```python
from build123d import *

# Parameters (mm, degrees)
ESTRUSIONE_ESTRUSIONE1_DEPTH = 2.5
SCHIZZO2_W                   = 10
SCHIZZO2_H                   = 38
ESTRUSIONE_ESTRUSIONE2_DEPTH = 15
SCHIZZO3_W                   = 6
SCHIZZO3_H                   = 33.15
TAGLIO_ESTRUSIONE1_DEPTH     = 20
ESTRUSIONE_SOTTILE1_START    = 19
SCHIZZO5_R                   = 21
SCHIZZO5_R_2                 = 18
ESTRUSIONE_SOTTILE1_DEPTH    = 19
SCHIZZO8_W                   = 38
SCHIZZO8_H                   = 15
TAGLIO_ESTRUSIONE2_DEPTH     = 70.157520353
SCHIZZO10_R                  = 3
ESTRUSIONE_ESTRUSIONE3_DEPTH = 4
FORO_PER_VITE_M1_6_1_D       = 2
FORO_PER_VITE_M1_6_1_DEPTH   = 3
FORO_PER_VITE_M1_6_1_TIP     = 0.600860619
SCHIZZO12_R                  = 1
TAGLIO_ESTRUSIONE3_DEPTH     = 3
FORO_PER_VITE_M3_1_D         = 3.6
FORO_PER_VITE_M3_1_DEPTH     = 4
FORO_PER_VITE_M3_1_TIP       = 1.081549114


with BuildPart() as part:
    # Schizzo1 → Estrusione-Estrusione1 (new, symmetric)
    with BuildSketch(Plane.XY):
        with BuildLine():
            Line((12.36549987, -26.390648792), (47.36549987, -26.390648792))
            Line((47.36549987, -26.390648792), (47.36549987, 11.609351208))
            Line((47.36549987, 11.609351208), (12.36549987, 11.609351208))
            ThreePointArc((12.36549987, 11.609351208), (-17.57877204, -7.390648792), (12.36549987, -26.390648792))
        make_face()
    extrude(amount=ESTRUSIONE_ESTRUSIONE1_DEPTH, both=True)

    # Schizzo2 → Estrusione-Estrusione2 (add)
    with BuildSketch(Plane.XY.offset(2.5)):
        with Locations((42.36549987, -7.390648792)):
            Rectangle(SCHIZZO2_W, SCHIZZO2_H)
    extrude(amount=ESTRUSIONE_ESTRUSIONE2_DEPTH)

    # Schizzo3 → Taglio-Estrusione1 (cut)
    with BuildSketch(Plane.XY.offset(17.5)):
        with Locations((42.36549987, -8.315648792)):
            Rectangle(SCHIZZO3_W, SCHIZZO3_H)
    extrude(amount=-TAGLIO_ESTRUSIONE1_DEPTH, mode=Mode.SUBTRACT)

    # Schizzo5 → Estrusione-Sottile1 (add)
    with BuildSketch(Plane.XY.offset(2.5).offset(ESTRUSIONE_SOTTILE1_START)):
        with Locations((3.42122796, -7.390648792)):
            Circle(SCHIZZO5_R)
        with Locations((3.42122796, -7.390648792)):
            Circle(SCHIZZO5_R_2, mode=Mode.SUBTRACT)
    extrude(amount=-ESTRUSIONE_SOTTILE1_DEPTH)

    # Schizzo8 → Taglio-Estrusione2 (cut, through all)
    with BuildSketch(Plane(origin=(-4.406906628, 12.10787645, 0), x_dir=(0.9396926207859102, 0.3420201433256638, 0), z_dir=(-0.3420201433256638, 0.9396926207859102, 0))):
        with Locations((0.687151909, -10)):
            Rectangle(SCHIZZO8_W, SCHIZZO8_H)
    extrude(amount=-TAGLIO_ESTRUSIONE2_DEPTH, mode=Mode.SUBTRACT)

    # Schizzo10 → Estrusione-Estrusione3 (add)
    with BuildSketch(Plane.XY.offset(21.5)):
        with Locations((-11.482021075, 7.404389842)):
            Circle(SCHIZZO10_R)
        with Locations((18.324476995, -22.185687427)):
            Circle(SCHIZZO10_R)
        with Locations((-11.373810674, -22.293897828)):
            Circle(SCHIZZO10_R)
        with Locations((6.992461631, 13.303463657)):
            Circle(SCHIZZO10_R)
    extrude(amount=-ESTRUSIONE_ESTRUSIONE3_DEPTH)

    # Foro per Vite M1.6-1
    with Locations(Plane(origin=(6.992461631, 13.303463657, 21.5), x_dir=(1, 0, 0), z_dir=(0, 0, 1))):
        with Locations((0, 0), (-18.474482706, -5.899073815), (-18.366272305, -35.597361485), (11.332015364, -35.489151084)):
            Hole(FORO_PER_VITE_M1_6_1_D / 2, depth=FORO_PER_VITE_M1_6_1_DEPTH)
            with Locations((0, 0, -(FORO_PER_VITE_M1_6_1_DEPTH + FORO_PER_VITE_M1_6_1_TIP / 2))):  # 118° drill point
                Cone(0, FORO_PER_VITE_M1_6_1_D / 2, FORO_PER_VITE_M1_6_1_TIP, mode=Mode.SUBTRACT)

    # Schizzo12 → Taglio-Estrusione3 (cut)
    with BuildSketch(Plane.XY.offset(2.5)):
        with Locations((3.42122796, -7.390648792)):
            Circle(SCHIZZO12_R)
    extrude(amount=-TAGLIO_ESTRUSIONE3_DEPTH, mode=Mode.SUBTRACT)

    # Foro per Vite M3-1
    with Locations(Plane(origin=(42.36549987, 11.609351208, 7.5), x_dir=(1, 0, 0), z_dir=(0, 1, 0))):
        with Locations((0, 0)):
            Hole(FORO_PER_VITE_M3_1_D / 2, depth=FORO_PER_VITE_M3_1_DEPTH)
            with Locations((0, 0, -(FORO_PER_VITE_M3_1_DEPTH + FORO_PER_VITE_M3_1_TIP / 2))):  # 118° drill point
                Cone(0, FORO_PER_VITE_M3_1_D / 2, FORO_PER_VITE_M3_1_TIP, mode=Mode.SUBTRACT)


solid = part.part
```
Geometry check sheet. Reference: the model listing, model coordinates, mm. A direction names the side the tool comes from. Give positions to 0.01 mm unless a question says otherwise; leave off trailing zeros. Write each loop counter-clockwise with the first axis right and the second up, starting at its lowest first coordinate (ties: lowest second). Pieces come first, ordered by that corner, then holes.
1) Access from +Z, -Z, +X, -X, +Y, -Y to the whole of each face (thin tool, end or side, straight path). Record for faces 4 (the flat face through (21.23, -0.77, 10.1)), 5 (the flat face through (-14.476, -13.771, 10.105)), 6 (the flat face through (37, -26.391, 1)), 7 (the flat face through (45.365, -9, 8)), 8 (the cylindrical face through (3.96, -6.55, 1.02)).
2) Release check for a two-part mould opening along Z. For faces 1 (the cylindrical face through (6.531, 12.416, 19.979)), 2 (the cylindrical face through (41.535, 9.911, 9.097)), 3 (the conical face through (-11.28, -22.147, 18.003)) record: pulls with the +Z half, pulls with the -Z half, needs draft (parallel to the pull), parting line crosses it, or undercut.
3) Section check C-C, the plane x = -2. Record the boundary of the cut face in (y, z).
4) Section check B-B, the plane z = 7.5. Record the boundary of the cut face in (x, y), and give its area (3 significant figures).
5) Section check A-A, the plane z = 4.5. Record the boundary of the cut face in (x, y).
6) Material ranges on L1, parallel to X at y = 8, z = 16; L2, parallel to Z at x = 10, y = -24.5; L3, parallel to X at y = 9.75, z = 7.5, recorded low to high.
7) Section check D-D, the plane x = 27. Record the boundary of the cut face in (y, z).
8) Gauge pin test, flat ends, axial feed: pin 1 (3 mm diameter, centred on x = 40, z = 4, fed in from -Y); pin 2 (8 mm diameter, centred on y = 11.5, z = 1.5, fed in from -X); pin 3 (5 mm diameter, centred on x = 41, z = 9, fed in from +Y). Record the tip position at first contact, or that the pin passes through.
Computed:
1. face 4: -Y
1. face 5: +Y
1. face 6: +Z, -Z, +X, -Y
1. face 7: +Z, -Z
1. face 8: +Z
2. face 1: needs draft
2. face 2: undercut
2. face 3: pulls with the +Z half
3. outline: (-27.68, -2.5) - (12.9, -2.5) - (12.9, 2.5) - (-27.68, 2.5) - close; (-27.68, 17.5) - (-24.55, 17.5) - (-24.55, 21.5) - (-27.68, 21.5) - close; (9.77, 17.5) - (12.9, 17.5) - (12.9, 21.5) - (9.77, 21.5) - close
4. outline: (-17.49, -5.48) arc R21 ccw to (-11.37, -22.29) - close; (18.22, 7.51) - (24.33, -9.3) arc R21 ccw to start; (37.37, -26.39) - (47.37, -26.39) - (47.37, 11.61) - (44.17, 11.61) - (44.17, 8.26) - (45.37, 8.26) - (45.37, -24.89) - (39.37, -24.89) - (39.37, 8.26) - (40.57, 8.26) - (40.57, 11.61) - (37.37, 11.61) - close
4. area: 217 mm2
5. outline: (-17.49, -5.48) arc R21 ccw to (-11.37, -22.29) - close; (18.22, 7.51) - (24.33, -9.3) arc R21 ccw to start; (37.37, -26.39) - (47.37, -26.39) - (47.37, 11.61) - (37.37, 11.61) - close; hole (39.37, -24.89) - (45.37, -24.89) - (45.37, 8.26) - (39.37, 8.26) - close
6. L1: x = 37.37 to 39.37, 45.37 to 47.37
6. L2: z = -2.5 to 2.5, 17.5 to 21.5
6. L3: x = 37.37 to 40.57, 44.17 to 47.37
7. outline: (-26.39, -2.5) - (11.61, -2.5) - (11.61, 2.5) - (-26.39, 2.5) - close
8. pin 1: stops at y = -26.39
8. pin 2: stops at x = -11.39
8. pin 3: stops at y = 11.61
